Study the drawing (mm; zero at the part's minimum x, y, z) and answer. Coordinates: 2 decimals unless noted, no trailing zeros. Loops run counter-clockwise (first coordinate to the right, second up) from the corner with the lowest first, then second, coordinate; pieces in that order, holes last. Notation, with made-up numbers: (56, 13) -> (67, 13) arc R14 cw to (67, 30) -> close; hole circle Ø11 at (-28, -0.5). An arc over 180 degrees is marked (long way). Answer as a JSON object with one key per item and string values. Group by question number.
Q1. Each of these flat-tipped pins is pushed along its axis until it touches: P1, Ø12, axis at y = 97, z = 32, coming from the -X side; P2, Ø3.5, axis at x = 5, y = 113.5, coming from the +Z side; P3, Ø2, axis at x = 4.5, z = 1.5, coming from the -Y side. Where does it stop, or does it pass through?
Q2. The part is cut by section C-C on y = 112.5. Write down the section's boundary in (x, z).
Q3. The part is cut by section A-A on z = 80. Write down the section's boundary in (x, y).
Q4. Straight lines are drawn through the part: line 1 along Y through (x, z) = (5, 2.85); line 2 along X through (y, z) = (112.5, 2.6); line 3 along X through (y, z) = (100.5, 42). For each, find the intervals that lie inside material, in ascending order. Write a range as [from, to].
Q5. The part is cut by section B-B on x = 5. Write down the section's boundary in (y, z).
Q6. The part is cut by section D-D on z = 54. Write down the section's boundary in (x, y), and give its area (3 significant figures).
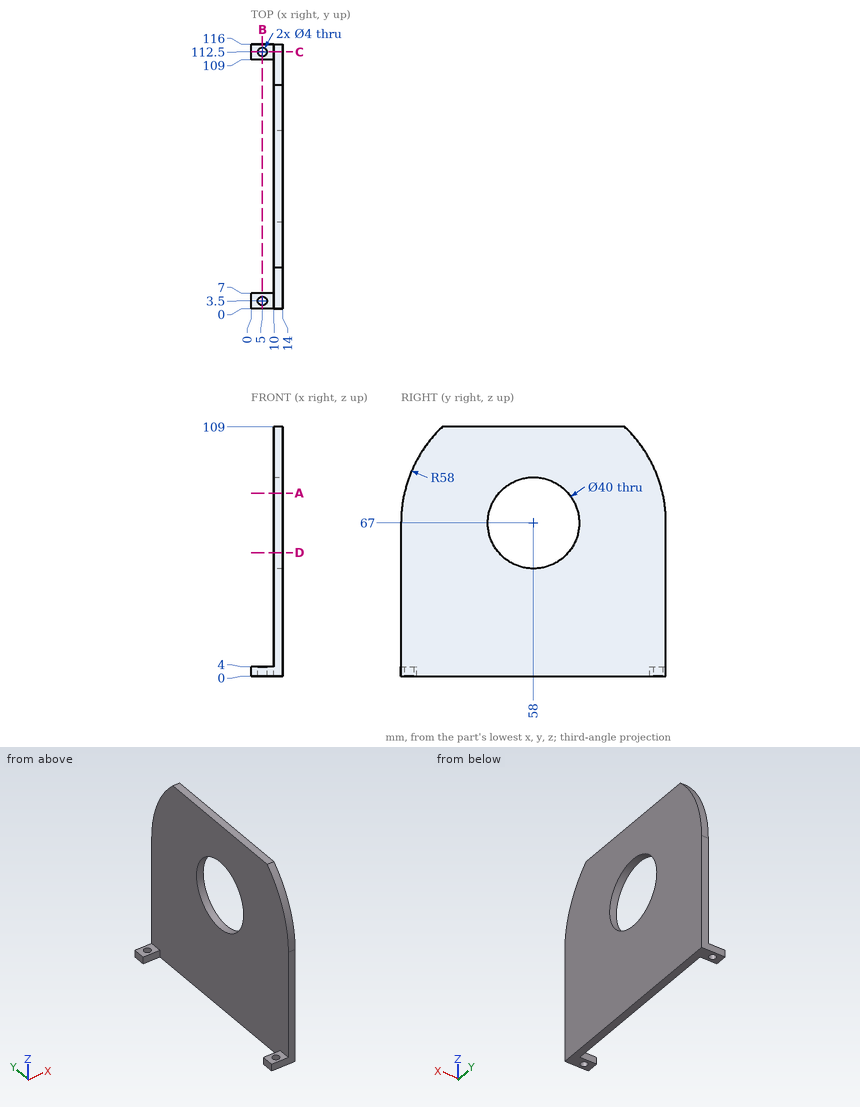
Final values:
{
 "1": {"P1": "stops at x = 10", "P2": "stops at z = 4", "P3": "stops at y = 0"},
 "2": {"outline": "(0, 0) -> (3, 0) -> (3, 4) -> (0, 4) -> close; (7, 0) -> (14, 0) -> (14, 86.84) -> (10, 86.84) -> (10, 4) -> (7, 4) -> close"},
 "3": {"outline": "(10, 1.48) -> (14, 1.48) -> (14, 42.8) -> (10, 42.8) -> close; (10, 73.2) -> (14, 73.2) -> (14, 114.52) -> (10, 114.52) -> close"},
 "4": {"line 1": "y = [0, 1.5], [5.5, 7], [109, 110.5], [114.5, 116]", "line 2": "x = [0, 3], [7, 14]", "line 3": "x = [10, 14]"},
 "5": {"outline": "(0, 0) -> (1.5, 0) -> (1.5, 4) -> (0, 4) -> close; (5.5, 0) -> (7, 0) -> (7, 4) -> (5.5, 4) -> close; (109, 0) -> (110.5, 0) -> (110.5, 4) -> (109, 4) -> close; (114.5, 0) -> (116, 0) -> (116, 4) -> (114.5, 4) -> close"},
 "6": {"outline": "(10, 0) -> (14, 0) -> (14, 42.8) -> (10, 42.8) -> close; (10, 73.2) -> (14, 73.2) -> (14, 116) -> (10, 116) -> close", "area": "342 mm2"}
}
